Build history of the part. All positions in model axes, mm. A direction names the side the tool comes from. Coordinates: 2 decimals unless noted, no trailing zeros. Loops run counter-clockwise (first coordinate to the right, second up) from the corner with the lowest first, then second, coordinate; pieces in that order, holes last.
(1) Slice it at B-B (y = -19). Give the cut face in (x, z) (3 decimals), and give its area (3 significant figures).
(2) Slice it at A-A (z = 0). Give the cut face in (x, y) (3 decimals).
(3) Two-plate mould, pull along Y, no slides. Class faces 4 (the face through (-14, -2, 0)), 5 (the face through (0, -14.18, -6)), 6 (the face through (-19.185, -14, 0)): pulls with the +Y half, pulls with the -Y half, needs draft (parallel to the pull), parting line crosses it, or undercut.
(4) Wall check: L1, parallel to Z at x = 0, y = -22.5; L2, parallel to Z at x = 0, y = -19; L3, parallel to Y at x = 1.5, z = 7. Give the ranges that are in metal, low to high.
(5) Flat gauge pins, fed straight in: P1, Ø5, axis at x = -12.5, y = -20, coming from the -Z side; P2, Ø9, axis at x = -9, z = -9, coming from the +Y side; P3, Ø13, axis at x = -5.5, y = -26, coming from the +Z side. Where does each tip first touch, or does it go through?
(6) Slice it at D-D (y = 24.5). Give the cut face in (x, z) (3 decimals).
(7) Slice it at C-C (x = -7.5). Give the cut face in (y, z) (3 decimals).
(8) Tool access for faces 1 (the face through (0, -7, 15)), 2 (the face through (-0.23, -23.31, -3.87)), 3 (the face through (3, 32.43, 3)): list every direction of +Z, -Z, +X, -X, +Y, -Y with a clear straight run to the whole face (end or side of a thin tool).
from build123d import *

# Parameters (mm, degrees)
SKETCH1_R                = 15.595
BOSS_EXTRUDE1_DEPTH      = 32.43
SKETCH2_R                = 4
BOSS_EXTRUDE2_DEPTH      = 3.7
SKETCH3_W                = 28
SKETCH3_H                = 30
BOSS_EXTRUDE3_DEPTH      = 14.18
SKETCH5_R                = 11.375
BOSS_EXTRUDE4_DEPTH      = 19.185
BOSS_EXTRUDE4_DEPTH_BACK = 19.185
SKETCH7_W                = 24.6
SKETCH7_H                = 19
BOSS_EXTRUDE5_DEPTH      = 18
SKETCH8_R                = 1.74191559
CUT_EXTRUDE1_DEPTH       = 18


with BuildPart() as part:
    # Sketch1 → Boss-Extrude1 (new body)
    with BuildSketch(Plane(origin=(0, 0, 0), x_dir=(1, 0, 0), z_dir=(0, 1, 0))):
        Circle(SKETCH1_R)
    extrude(amount=BOSS_EXTRUDE1_DEPTH)

    # Sketch2 → Boss-Extrude2 (add)
    with BuildSketch(Plane(origin=(0, 32.43, 0), x_dir=(1, 0, 0), z_dir=(0, 1, 0))):
        Circle(SKETCH2_R)
    extrude(amount=BOSS_EXTRUDE2_DEPTH)

    # Sketch3 → Boss-Extrude3 (add)
    with BuildSketch(Plane.XZ):
        Rectangle(SKETCH3_W, SKETCH3_H)
    extrude(amount=BOSS_EXTRUDE3_DEPTH)

    # Sketch5 → Boss-Extrude4 (add, two sides)
    with BuildSketch(Plane.ZY) as boss_extrude4_sk:
        with Locations((0, -14.18)):
            Circle(SKETCH5_R)
    extrude(amount=BOSS_EXTRUDE4_DEPTH)
    extrude(boss_extrude4_sk.sketch, amount=-BOSS_EXTRUDE4_DEPTH_BACK)

    # Sketch7 → Boss-Extrude5 (add)
    with BuildSketch(Plane.XZ.offset(14.18)):
        Rectangle(SKETCH7_W, SKETCH7_H)
    extrude(amount=BOSS_EXTRUDE5_DEPTH)

    # Sketch8 → Cut-Extrude1 (cut)
    with BuildSketch(Plane.XZ.offset(32.18)):
        with Locations((0, 5.595)):
            Circle(SKETCH8_R)
        with Locations((0, -5.595)):
            Circle(SKETCH8_R)
    extrude(amount=-CUT_EXTRUDE1_DEPTH, mode=Mode.SUBTRACT)


solid = part.part
Response values:
1. outline: (-19.185, -10.303) - (19.185, -10.303) - (19.185, 10.303) - (-19.185, 10.303) - close; hole circle Ø3.484 at (0, -5.595); hole circle Ø3.484 at (0, 5.595)
1. area: 772 mm2
2. outline: (-19.185, -25.555) - (-12.3, -25.555) - (-12.3, -32.18) - (12.3, -32.18) - (12.3, -25.555) - (19.185, -25.555) - (19.185, -2.805) - (14, -2.805) - (14, 0) - (15.595, 0) - (15.595, 32.43) - (4, 32.43) - (4, 36.13) - (-4, 36.13) - (-4, 32.43) - (-15.595, 32.43) - (-15.595, 0) - (-14, 0) - (-14, -2.805) - (-19.185, -2.805) - close
3. face 4: undercut
3. face 5: pulls with the -Y half
3. face 6: needs draft
4. L1: z = -9.5 to -7.34, -3.85 to 3.85, 7.34 to 9.5
4. L2: z = -10.3 to -7.34, -3.85 to 3.85, 7.34 to 10.3
4. L3: y = -32.18 to 32.43
5. P1: stops at z = -10.88
5. P2: stops at y = 32.43
5. P3: stops at z = 10.05
6. outline: circle Ø31.19 at (0, 0)
7. outline: (-32.18, -9.5) - (-20.436, -9.5) arc R11.375 ccw to (-14.18, -11.375) - (-14.18, -15) - (0, -15) - (0, -13.673) - (32.43, -13.673) - (32.43, 13.673) - (0, 13.673) - (0, 15) - (-14.18, 15) - (-14.18, 11.375) arc R11.375 ccw to (-20.436, 9.5) - (-32.18, 9.5) - close
8. face 1: +Z, +X, -X, -Y
8. face 2: -Y
8. face 3: +Y
